from build123d import *

# Parameters (mm, degrees)
BOSS_EXTRUDE3_DEPTH      = 25
SKETCH5_R                = 7
BOSS_EXTRUDE4_DEPTH      = 20
BOSS_EXTRUDE6_REACH      = 91.582
BOSS_EXTRUDE6_END_RADIUS = 40
SKETCH8_W                = 40
SKETCH8_H                = 30
SKETCH9_W                = 30
SKETCH9_H                = 20
CUT_EXTRUDE3_DEPTH       = 10
SKETCH10_R               = 7.5
CUT_EXTRUDE4_DEPTH       = 90.582364336


with BuildPart() as part:
    # Sketch4 → Boss-Extrude3 (new, symmetric)
    with BuildSketch(Plane.XY):
        with BuildLine():
            Line((-34.580398915, 5), (-29.580398915, 5))
            ThreePointArc((-29.580398915, 5), (0, 30), (29.580398915, 5))
            Line((29.580398915, 5), (34.580398915, 5))
            Line((34.580398915, 5), (34.580398915, 0))
            Line((34.580398915, 0), (40, 0))
            ThreePointArc((40, 0), (0, 40), (-40, 0))
            Line((-40, 0), (-34.580398915, 0))
            Line((-34.580398915, 0), (-34.580398915, 5))
        make_face()
    extrude(amount=BOSS_EXTRUDE3_DEPTH, both=True)

    # Sketch5 → Boss-Extrude4 (add)
    # profile 1 of 2: a face of its own
    with BuildSketch(Plane(origin=(0, 0, 0), x_dir=(1, 0, 0), z_dir=(0, 1, 0))):
        with BuildLine():
            Line((-55, 15), (-34.580398915, 15))
            Line((-34.580398915, 15), (-34.580398915, -15))
            Line((-34.580398915, -15), (-55, -15))
            ThreePointArc((-55, -15), (-70, 0), (-55, 15))
        make_face()
        with Locations(Location((-55, 0, 0), (0, 0, 270))):
            Circle(SKETCH5_R, mode=Mode.SUBTRACT)
    # profile 2 of 2: a face of its own
    with BuildSketch(Plane(origin=(0, 0, 0), x_dir=(1, 0, 0), z_dir=(0, 1, 0))):
        with BuildLine():
            Line((34.580398915, 15), (55, 15))
            ThreePointArc((55, 15), (70, 0), (55, -15))
            Line((55, -15), (34.580398915, -15))
            Line((34.580398915, -15), (34.580398915, 15))
        make_face()
        with Locations(Location((55, 0, 0), (0, 0, 270))):
            Circle(SKETCH5_R, mode=Mode.SUBTRACT)
    extrude(amount=BOSS_EXTRUDE4_DEPTH)

    # Boss-Extrude6: up to this cylinder (the profile starts outside it)
    boss_extrude6_end = Plane(origin=(0, 0, 0), z_dir=(0, 0, -1)) * Cylinder(BOSS_EXTRUDE6_END_RADIUS, 264.164, mode=Mode.PRIVATE)
    # Sketch8 → Boss-Extrude6 (add, up to the surface)
    with BuildSketch(Plane(origin=(0, 50, 0), x_dir=(1, 0, 0), z_dir=(0, 1, 0)), mode=Mode.PRIVATE) as boss_extrude6_sk1:
        Rectangle(SKETCH8_W, SKETCH8_H)
    boss_extrude6_tool1 = extrude(boss_extrude6_sk1.sketch, amount=-BOSS_EXTRUDE6_REACH, mode=Mode.PRIVATE) - boss_extrude6_end
    add(boss_extrude6_tool1.solids().sort_by_distance((0, 50, 0))[0])

    # Sketch9 → Cut-Extrude3 (cut)
    with BuildSketch(Plane(origin=(0, 50, 0), x_dir=(1, 0, 0), z_dir=(0, 1, 0))):
        Rectangle(SKETCH9_W, SKETCH9_H)
    extrude(amount=-CUT_EXTRUDE3_DEPTH, mode=Mode.SUBTRACT)

    # Sketch10 → Cut-Extrude4 (cut, through all)
    with BuildSketch(Plane(origin=(0, 50, 0), x_dir=(1, 0, 0), z_dir=(0, 1, 0))):
        with Locations(Location((0, 0, 0), (0, 0, 270))):
            Circle(SKETCH10_R)
    extrude(amount=-CUT_EXTRUDE4_DEPTH, mode=Mode.SUBTRACT)


solid = part.part
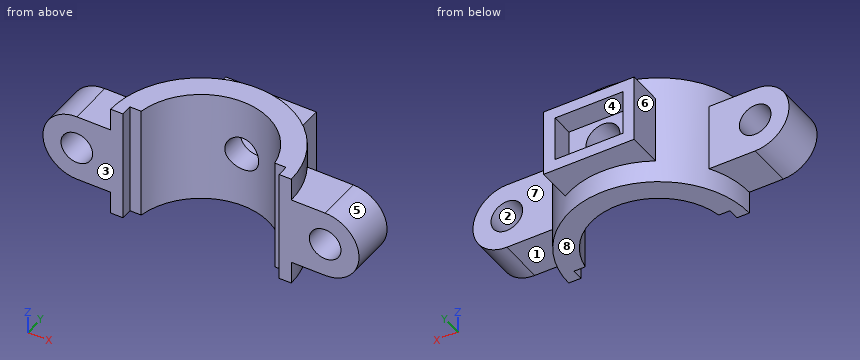
Model file for the job. Use its own axes, mm. Face numbers are marked on the shaded views. A direction names the side the tool comes from. Give positions to 0.01 mm unless a question says otherwise; leave off trailing zeros. Write each loop counter-clockwise with the first axis right and the second up, starting at its lowest first coordinate (ties: lowest second). Pieces come first, ordered by that corner, then holes. Notation, with made-up numbers: (-3, 34.25) - (51, 34.25) arc R12 ccw to (51, 51.25) - close; hole circle Ø3 at (43.25, 40). An arc over 180 degrees is marked (long way). Answer as CSV lines item,"result".
1. Two-plate mould, pull along Z, no slides. Class the marked faces 1, 2 and 3: +Z half, -Z half, draft (parallel to the pull), parting line (faces both ways), or undercut.
Responses:
face 1,"-Z half"
face 2,"undercut"
face 3,"draft"
2. Pin check, flat tips, straight feed: pin 1 (3 mm diameter, centred on y = 43.5, z = -1.5, fed in from +X); pin 2 (10 mm diameter, centred on x = 47.5, y = 12, fed in from -Z); pin 3 (6 mm diameter, centred on x = -5.5, z = 17.5, fed in from -Y); pin 4 (24 mm diameter, centred on x = 0, z = 0, fed in from +Y). Stop position of each tip, or through.
Responses:
pin 1,"stops at x = 20"
pin 2,"stops at z = -15"
pin 3,"stops at y = 28.77"
pin 4,"stops at y = 50"
3. Band-saw the part on A-A (x = 0). Write the cut outline in (y, z), and give its area (3 significant figures).
Responses:
outline,"(30, -25) - (40, -25) - (40, -15) - (50, -15) - (50, -10) - (40, -10) - (40, -7.5) - (30, -7.5) - close; (30, 7.5) - (40, 7.5) - (40, 10) - (50, 10) - (50, 15) - (40, 15) - (40, 25) - (30, 25) - close"
area,"450 mm2"
4. Band-saw the part on C-C (y = 31.5). Write the cut outline in (x, z), and give its area (3 significant figures).
Responses:
outline,"(-24.65, -25) - (24.65, -25) - (24.65, 25) - (-24.65, 25) - close; hole circle Ø15 at (0, 0)"
area,"2,290 mm2"
5. 3-axis set-ups, long thin cutter, end or side, ignore diameter. For the marked faces 4, 5, 6, 7 and 8: which of +Z, -Z, +X, -X, +Y, -Y reach the whole face in a straight line?
Responses:
face 4,"+Y"
face 5,"+X, +Y, -Y"
face 6,"+Z, -Z, -X, +Y"
face 7,"+Z, -Z, +X, +Y"
face 8,"-Z, +X, -X, +Y, -Y"
6. Band-saw the part on D-D (z = 11.5). Write the cut outline in (x, y).
Responses:
outline,"(-64.63, 0) - (-34.58, 0) - (-34.58, 5) - (-29.58, 5) arc R30 cw to (29.58, 5) - (34.58, 5) - (34.58, 0) - (64.63, 0) - (64.63, 20) - (34.64, 20) arc R40 ccw to (20, 34.64) - (20, 50) - (-20, 50) - (-20, 34.64) arc R40 ccw to (-34.64, 20) - (-64.63, 20) - close"
7. Band-saw the part on B-B (z = 0). Count the separate pieces of the cut face and the enclosed holes in it, and give its area (3 significant figures).
Responses:
separate pieces,"4"
enclosed holes,"0"
area,"1,780 mm2"
8. Drill centre lines: L1, parallel to X at y = 4, z = 0; L2, parallel to X at y = 14.5, z = 0; L3, parallel to Z at x = 0, y = 36.5. Where is each one in solid material? Low to high. Write a range as [from, to].
Responses:
L1,"x = [-70, -62], [-48, -34.58], [34.58, 48], [62, 70]"
L2,"x = [-70, -62], [-48, -26.26], [26.26, 48], [62, 70]"
L3,"z = [-25, -7.5], [7.5, 25]"
